Geometry: final body of the model. Coordinates: model frame, mm. Round coordinates to 2 decimals unless told otherwise and drop trailing zeros. Order: outer loops, then holes, each group sorted by start corner. A loop starts at its lowest first (then second) coordinate and runs counter-clockwise, first axis right, second up. Notation, with made-up numbers: (64, 21.5) -> (112, 21.5) arc R21 cw to (112, 44.5) -> close; hole circle Ø6 at (-24.5, 22.25). An arc over 180 degrees is marked (long way). Put each result on its own line as item: value.
```python
from build123d import *

# Parameters (mm, degrees)
SKETCH1_R           = 1
BOSS_EXTRUDE1_DEPTH = 4


with BuildPart() as part:
    # Sketch1 → Boss-Extrude1 (new body)
    with BuildSketch(Plane.XY):
        with BuildLine():
            Line((-14.257280668, -1.575118781), (-14.828930549, -0.86376259))
            ThreePointArc((-14.828930549, -0.86376259), (-14.717335158, 1.065944375), (-13.025069638, 2))
            Line((-13.025069638, 2), (7.597126091, 7.882366595))
            ThreePointArc((7.597126091, 7.882366595), (11.968265738, 7.707732331), (15.382140621, 4.972258475))
            Line((15.382140621, 4.972258475), (18.503191116, 0.182221363))
            ThreePointArc((18.503191116, 0.182221363), (18.275196012, -1.064934274), (17.471757811, -2.045681953))
            Line((17.471757811, -2.045681953), (2.208569451, -7.726919547))
            ThreePointArc((2.208569451, -7.726919547), (-2.503379707, -8.279944918), (-6.939921558, -6.599052796))
            Line((-6.939921558, -6.599052796), (-14.257280668, -1.575118781))
        make_face()
        with Locations((15.974930362, 0)):
            Circle(SKETCH1_R, mode=Mode.SUBTRACT)
        with Locations((-13.025069638, 0)):
            Circle(SKETCH1_R, mode=Mode.SUBTRACT)
    extrude(amount=BOSS_EXTRUDE1_DEPTH)


solid = part.part
```
1. Cut plane A-A on z = 1.25. Return loops of the section in (x, y).
Ans:
outline: (-14.83, -0.86) -> (-14.26, -1.58) -> (-6.94, -6.6) arc R10 ccw to (2.21, -7.73) -> (17.47, -2.05) arc R2.53 ccw to (18.5, 0.18) -> (15.38, 4.97) arc R7 ccw to (7.6, 7.88) -> (-13.03, 2) arc R2 ccw to start; hole circle Ø2 at (-13.03, 0); hole circle Ø2 at (15.97, 0)
2. Contact query for flat-ended pins moving along their axis: P1, Ø1.5, axis at x = -7.5, z = 3.5, coming from the +Y side; P2, Ø2, axis at x = 13, z = 2, coming from the +Y side. Output: stop coordinate, or through.
Ans:
P1: y = 3.79
P2: y = 7.7
3. Cut plane B-B on x = -1.5. Return loops of the section in (y, z).
Ans:
outline: (-8.35, 0) -> (5.29, 0) -> (5.29, 4) -> (-8.35, 4) -> close
4. Cut plane C-C on y = 5.5. Return loops of the section in (x, z), and give its area (3 significant figures).
Ans:
outline: (-0.75, 0) -> (15, 0) -> (15, 4) -> (-0.75, 4) -> close
area: 63.0 mm²
5. Material intervals for probe 1 along Y at (x, z) = (16, 2.55); probe 2 along Y at (x, z) = (5, 2.55); probe 3 along Y at (x, z) = (5.5, 1.95), sorted ascending.
Ans:
probe 1: -2.59 to -1, 1 to 4.02
probe 2: -6.69 to 7.14
probe 3: -6.5 to 7.28
6. Draft query along X for faces 1 (the face through (-14.732, 1.042, 1.972)), 2 (the face through (-2.437, -8.288, 1.972)), 3 (the face through (-12.1, -0.38, 1.97)), 4 (the face through (9.947, -4.847, 1.972)). Return one class per face: +X half, -X half, draft (parallel to the pull), parting line (faces both ways), or undercut.
Ans:
face 1: -X half
face 2: parting line
face 3: undercut
face 4: +X half
